Verification items for this drawing (mm, ordinates from the low corner). A direction names the side the tool comes from. Give positions to 0.01 mm unless a question says otherwise; leave off trailing zeros. Order: outer loops, then holes, each group sorted by start corner. A loop starts at its lowest first (then second) coordinate and runs counter-clockwise, first axis right, second up. Notation, with made-up numbers: (51.25, 83.5) - (82.25, 83.5) arc R12 ccw to (82.25, 98.5) - close; hole circle Ø6 at (28.25, -13). An arc over 180 degrees is marked (long way). Put each result on its own line as item: value. Start each with the question number.
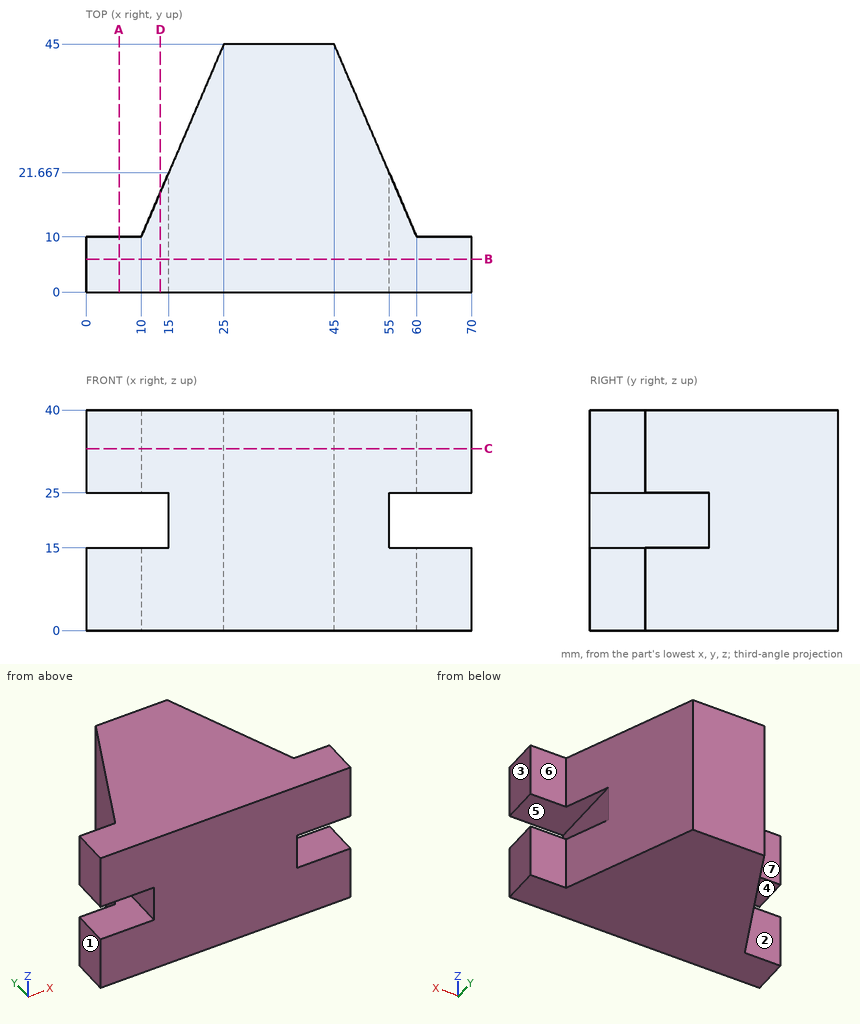
Item 1: Cross-section at C-C (z = 33). Enter the section's corners in (x, y), and give its area (4 significant figures).
Item 2: Cross-section at B-B (y = 6). Enter the section's corners in (x, z), and give its area (3 significant figures).
Item 3: Set-up check for the marked faces 4, 5, 6 and 7: record each of +Z, -Z, +X, -X, +Y, -Y from which the full face is reachable in a straight line by a thin tool's end or side.
Item 4: Thickness scan on line 1 along Z through (x, y) = (7, 4); line 2 along Y through (x, z) = (67, 13); line 3 along X through (y, z) = (17, 21). Record the ranges inside material, lowest first.
Item 5: Cross-section at D-D (x = 13.5). Enter the section's corners in (y, z).
Item 6: Cross-section at A-A (x = 6). Enter the section's corners in (y, z).
Item 7: Release check for a two-part mould opening along X. For the marked faces 1, 2 and 3 record: +X half, -X half, draft (parallel to the pull), parting line (faces both ways), or undercut.
Item 8: Gauge pin test, flat ends, axial feed: pin 1 Ø5 at (x, z) = (5, 6) entering from +Y; pin 2 Ø5 at (y, z) = (15.5, 7) entering from +X (1 decimal); pin 3 Ø4.5 at (x, y) = (64.5, 12.5) entering from -Z; pin 4 Ø1 at (x, z) = (54, 25.5) entering from -Y. Record the tip position at first contact, or that the pin passes through.
Recorded:
1. outline: (0, 0) - (70, 0) - (70, 10) - (60, 10) - (45, 45) - (25, 45) - (10, 10) - (0, 10) - close
1. area: 1,925 mm^2
2. outline: (0, 0) - (70, 0) - (70, 15) - (55, 15) - (55, 25) - (70, 25) - (70, 40) - (0, 40) - (0, 25) - (15, 25) - (15, 15) - (0, 15) - close
2. area: 2,500 mm^2
3. face 4: -X, +Y, -Y
3. face 5: +X, +Y, -Y
3. face 6: +Z, -Z, +X, +Y
3. face 7: +Z, -Z, -X, +Y
4. line 1: z = 0 to 15, 25 to 40
4. line 2: y = 0 to 10
4. line 3: x = 15 to 55
5. outline: (0, 0) - (18.17, 0) - (18.17, 15) - (0, 15) - close; (0, 25) - (18.17, 25) - (18.17, 40) - (0, 40) - close
6. outline: (0, 0) - (10, 0) - (10, 15) - (0, 15) - close; (0, 25) - (10, 25) - (10, 40) - (0, 40) - close
7. face 1: -X half
7. face 2: draft
7. face 3: +X half
8. pin 1: stops at y = 10
8. pin 2: stops at x = 58.7
8. pin 3: passes through
8. pin 4: stops at y = 0
